```python
from build123d import *

# Parameters (mm, degrees)
SZKIC1_W                            = 27.5
SZKIC1_H                            = 200
SFAZOWANIE1_SIZE                    = 1
OTW_R_GWINTOWANY_M8X1_01_AT_2_COUNT = 2
OTW_R_GWINTOWANY_M8X1_01_AT_2_PITCH = 137.316
OTW_R_GWINTOWANY_M8X1_01_AT_3_COUNT = 2
OTW_R_GWINTOWANY_M8X1_01_AT_3_PITCH = 237.838288692
OTW_R_GWINTOWANY_M8X1_01_AT_4_COUNT = 2
OTW_R_GWINTOWANY_M8X1_01_AT_4_PITCH = 274.632
OTW_R_GWINTOWANY_M8X1_01_AT_5_COUNT = 2
OTW_R_GWINTOWANY_M8X1_01_AT_5_PITCH = 237.838288692
OTW_R_GWINTOWANY_M8X1_01_AT_6_COUNT = 2
OTW_R_GWINTOWANY_M8X1_01_AT_6_PITCH = 137.316


with BuildPart() as part:
    # Szkic1 → Obrót1 (revolve)
    with BuildSketch(Plane.XY):
        with Locations((-136.25, 73.59625624)):
            Rectangle(SZKIC1_W, SZKIC1_H)
    revolve(axis=Axis((0, 193.59625624, 0), (0, -1, 0)))

    # Sfazowanie1
    sfazowanie1_edges = [part.edges().sort_by_distance(p)[0] for p in [
        (150, 173.59625624, 0),
        (122.5, 173.59625624, 0),
        (122.5, -26.40374376, 0),
        (150, -26.40374376, 0),
    ]]
    chamfer(sfazowanie1_edges, length=SFAZOWANIE1_SIZE)

    # Szkic7 → Otwór gwintowany M8x1.01 (revolve, cut)
    with BuildSketch(Plane(origin=(0, 173.59625624, -137.316), x_dir=(0, 0, 1), z_dir=(1, 0, 0))):
        Polygon((0, 0), (0, 77.103012167), (3.5, 75), (3.5, 0), align=None)
    otw_r_gwintowany_m8x1_01 = revolve(axis=Axis((0, 179.94625624, -137.316), (0, -1, 0)), mode=Mode.SUBTRACT)

    # Otwór gwintowany M8x1.01 at 2: Otwór gwintowany M8x1.01 ×2
    with Locations(*[Vector(0.8660254037844388, 0, 0.49999999999999983) * (i * OTW_R_GWINTOWANY_M8X1_01_AT_2_PITCH) for i in range(1, OTW_R_GWINTOWANY_M8X1_01_AT_2_COUNT)]):
        add(otw_r_gwintowany_m8x1_01, mode=Mode.SUBTRACT)

    # Otwór gwintowany M8x1.01 at 3: Otwór gwintowany M8x1.01 ×2
    with Locations(*[Vector(0.5000000000000001, 0, 0.8660254037844386) * (i * OTW_R_GWINTOWANY_M8X1_01_AT_3_PITCH) for i in range(1, OTW_R_GWINTOWANY_M8X1_01_AT_3_COUNT)]):
        add(otw_r_gwintowany_m8x1_01, mode=Mode.SUBTRACT)

    # Otwór gwintowany M8x1.01 at 4: Otwór gwintowany M8x1.01 ×2
    with Locations(*[(0, 0, i * OTW_R_GWINTOWANY_M8X1_01_AT_4_PITCH) for i in range(1, OTW_R_GWINTOWANY_M8X1_01_AT_4_COUNT)]):
        add(otw_r_gwintowany_m8x1_01, mode=Mode.SUBTRACT)

    # Otwór gwintowany M8x1.01 at 5: Otwór gwintowany M8x1.01 ×2
    with Locations(*[Vector(-0.49999999999999967, 0, 0.8660254037844388) * (i * OTW_R_GWINTOWANY_M8X1_01_AT_5_PITCH) for i in range(1, OTW_R_GWINTOWANY_M8X1_01_AT_5_COUNT)]):
        add(otw_r_gwintowany_m8x1_01, mode=Mode.SUBTRACT)

    # Otwór gwintowany M8x1.01 at 6: Otwór gwintowany M8x1.01 ×2
    with Locations(*[Vector(-0.8660254037844386, 0, 0.5000000000000002) * (i * OTW_R_GWINTOWANY_M8X1_01_AT_6_PITCH) for i in range(1, OTW_R_GWINTOWANY_M8X1_01_AT_6_COUNT)]):
        add(otw_r_gwintowany_m8x1_01, mode=Mode.SUBTRACT)

    # Lustro2: Otwór gwintowany M8x1.01 across plane
    add(otw_r_gwintowany_m8x1_01.mirror(Plane.ZX.offset(73.59625624)), mode=Mode.SUBTRACT)

    # Lustro2 copy 1 sketch → Lustro2 copy 1 (revolve, cut)
    with BuildSketch(Plane(origin=(118.919144346, -26.40374376, -68.658), x_dir=(0, 0, 1), z_dir=(1, 0, 0))):
        Polygon((0, 0), (0, -77.103012167), (3.5, -75), (3.5, 0), align=None)
    revolve(axis=Axis((118.919144346, -32.75374376, -68.658), (0, -1, 0)), mode=Mode.SUBTRACT)

    # Lustro2 copy 2 sketch → Lustro2 copy 2 (revolve, cut)
    with BuildSketch(Plane(origin=(118.919144346, -26.40374376, 68.658), x_dir=(0, 0, 1), z_dir=(1, 0, 0))):
        Polygon((0, 0), (0, -77.103012167), (3.5, -75), (3.5, 0), align=None)
    revolve(axis=Axis((118.919144346, -32.75374376, 68.658), (0, -1, 0)), mode=Mode.SUBTRACT)

    # Lustro2 copy 3 sketch → Lustro2 copy 3 (revolve, cut)
    with BuildSketch(Plane(origin=(0, -26.40374376, 137.316), x_dir=(0, 0, 1), z_dir=(1, 0, 0))):
        Polygon((0, 0), (0, -77.103012167), (3.5, -75), (3.5, 0), align=None)
    revolve(axis=Axis((0, -32.75374376, 137.316), (0, -1, 0)), mode=Mode.SUBTRACT)

    # Lustro2 copy 4 sketch → Lustro2 copy 4 (revolve, cut)
    with BuildSketch(Plane(origin=(-118.919144346, -26.40374376, 68.658), x_dir=(0, 0, 1), z_dir=(1, 0, 0))):
        Polygon((0, 0), (0, -77.103012167), (3.5, -75), (3.5, 0), align=None)
    revolve(axis=Axis((-118.919144346, -32.75374376, 68.658), (0, -1, 0)), mode=Mode.SUBTRACT)

    # Lustro2 copy 5 sketch → Lustro2 copy 5 (revolve, cut)
    with BuildSketch(Plane(origin=(-118.919144346, -26.40374376, -68.658), x_dir=(0, 0, 1), z_dir=(1, 0, 0))):
        Polygon((0, 0), (0, -77.103012167), (3.5, -75), (3.5, 0), align=None)
    revolve(axis=Axis((-118.919144346, -32.75374376, -68.658), (0, -1, 0)), mode=Mode.SUBTRACT)


solid = part.part
```
The model under review builds one solid part; all positions refer to its coordinate system, in mm. Round coordinates to 2 decimals unless told otherwise and drop trailing zeros. Write each loop counter-clockwise with the first axis right and the second up, starting at its lowest first coordinate (ties: lowest second). Pieces come first, ordered by that corner, then holes.
(1) Wall thickness on L1, parallel to Z at x = 0, y = -4; L2, parallel to X at y = 119, z = 0: over which ranges is each line inside the solid? List them lowest first.
(2) Mouldability with a two-part tool opening along X and no side actions: class faces 1 (the cylindrical face through (26.556, 74.982, 119.587)), 2 (the flat face through (56, 173.596, -111)), 3 (the cylindrical face through (19.527, 74.982, -148.724)) as +X half, -X half, draft (parallel to the pull), parting line (faces both ways), or undercut.
(3) Insertion check: pin 1 (5 mm diameter, centred on x = 100, y = 115, fed in from -Z); pin 2 (4 mm diameter, centred on y = 74.5, z = -61, fed in from +X); pin 3 (5 mm diameter, centred on x = -90.5, y = 131.5, fed in from -Z). Each pin has a flat end and moves straight along its axis. Give the tip position at first contact, or say it passes through.
(4) We need section C-C on y = 9.5. Give the boundary of the cut face in (x, z).
(5) We need section B-B on y = 80.5. Give the boundary of the cut face in (x, z).
(6) We need section A-A on z = 0. Give the boundary of the cut face in (x, y), and give its area (3 significant figures).
Findings below:
1. L1: z = -150 to -140.82, -133.82 to -122.5, 122.5 to 133.82, 140.82 to 150
1. L2: x = -150 to -122.5, 122.5 to 150
2. face 1: undercut
2. face 2: draft
2. face 3: parting line
3. pin 1: stops at z = -113.99
3. pin 2: stops at x = 137.91
3. pin 3: stops at z = -121.47
4. outline: circle Ø300 at (0, 0); hole circle Ø245 at (0, 0); hole circle Ø7 at (-118.92, -68.66); hole circle Ø7 at (-118.92, 68.66); hole circle Ø7 at (0, -137.32); hole circle Ø7 at (0, 137.32); hole circle Ø7 at (118.92, -68.66); hole circle Ø7 at (118.92, 68.66)
5. outline: circle Ø300 at (0, 0); hole circle Ø245 at (0, 0)
6. outline: (-150, -25.4) - (-149, -26.4) - (-123.5, -26.4) - (-122.5, -25.4) - (-122.5, 172.6) - (-123.5, 173.6) - (-149, 173.6) - (-150, 172.6) - close; (122.5, -25.4) - (123.5, -26.4) - (149, -26.4) - (150, -25.4) - (150, 172.6) - (149, 173.6) - (123.5, 173.6) - (122.5, 172.6) - close
6. area: 11,000 mm2
